```python
from build123d import *

# Parameters (mm, degrees)
F2_SIZE = 0.1


with BuildPart() as f1:
    # F0 (on Right) → F1 (revolve)
    with BuildSketch(Plane.YZ):
        Polygon((-21.5, 2.25), (0, 2.25), (0, 4.5), (-0.8, 4.5), (-0.8, 4), (-1.6, 4), (-1.6, 4.5), (-2.4, 4.5), (-2.4, 3.5), (-13.7, 3.5), (-13.7, 3), (-20.5, 3), (-21.5, 2.5), align=None)
    revolve(axis=Axis((0, -10.75, 0), (0, -1, 0)))

    # F2
    f2_edges = [f1.edges().sort_by_distance(p)[0] for p in [
        (0, -13.7, -3.5),
    ]]
    chamfer(f2_edges, length=F2_SIZE)


solid = f1.part
```
Work out the finished part from the listing and answer in its coordinate system (mm). A direction names the side the tool comes from. Coordinates: 2 decimals unless noted, no trailing zeros. Write each loop counter-clockwise with the first axis right and the second up, starting at its lowest first coordinate (ties: lowest second). Pieces come first, ordered by that corner, then holes. Notation, with made-up numbers: (83.5, -30) - (130.5, -30) arc R14 ccw to (130.5, -17) - close; hole circle Ø2 at (73.25, 57.5). An arc over 180 degrees is marked (long way). Answer as a JSON object with one key per item and string values.
Q1. Which of the six approach directions +Z, -Z, +X, -X, +Y, -Y give full straight-line access (tool end or side, diameter ignored) to faces 1 (the cylindrical face through (0, -17, -3)), 2 (the flat face through (3, -1.6, 3)), 3 (the cylindrical face through (-4.46, -0.41, -0.59))?
Results list:
{"face 1": "-Y", "face 2": "none", "face 3": "+Y, -Y"}
Q2. Given pin 1 Ø1.5 at (x, z) = (3, 2) entering from -Y; pin 2 Ø1.5 at (y, z) = (-3.5, 0.5) entering from -X; pin 3 Ø4.5 at (x, z) = (-0.5, 2) entering from -Y; pin 4 Ø1.5 at (y, z) = (-13, 3) entering from +X, each flat-ended and moving along its own axis, determine where each tip first touches the part or whether it passes through.
Results list:
{"pin 1": "stops at y = -20.79", "pin 2": "stops at x = -3.5", "pin 3": "stops at y = -21.5", "pin 4": "stops at x = 2.68"}
Q3. For a pull along Z with two mould halves and no side action, classify faces 4 (the cylindrical face through (-4.46, -2.01, -0.59)), 5 (the flat face through (4, -2.4, 0)), 6 (the cylindrical face through (-2.23, -10.6, -0.29)) as pulls with the +Z half, pulls with the -Z half, needs draft (parallel to the pull), parting line crosses it, or undercut.
Results list:
{"face 4": "parting line crosses it", "face 5": "needs draft", "face 6": "undercut"}
Q4. Find section B-B (y = -7.25). Write down the section's boundary in (x, z), plus the area to 3 significant figures.
Results list:
{"outline": "circle Ø7 at (0, 0); hole circle Ø4.5 at (0, 0)", "area": "22.6 mm^2"}
Q5. Consider L1, parallel to Y at x = -2.75, z = 3.5; L2, parallel to X at y = -8.5, z = 0; L3, parallel to X at y = -16.75, z = 0. Determine where each line is inside the solid, lowest interval first. Write a range as from..to.
Results list:
{"L1": "y = -2.4..-1.6, -0.8..0", "L2": "x = -3.5..-2.25, 2.25..3.5", "L3": "x = -3..-2.25, 2.25..3"}
Q6. Find section C-C (y = -2). Write down the section's boundary in (x, z).
Results list:
{"outline": "circle Ø9 at (0, 0); hole circle Ø4.5 at (0, 0)"}
Q7. Find section A-A (z = 0). Write down the section's boundary in (x, y).
Results list:
{"outline": "(-4.5, -2.4) - (-3.5, -2.4) - (-3.5, -13.6) - (-3.4, -13.7) - (-3, -13.7) - (-3, -20.5) - (-2.5, -21.5) - (-2.25, -21.5) - (-2.25, 0) - (-4.5, 0) - (-4.5, -0.8) - (-4, -0.8) - (-4, -1.6) - (-4.5, -1.6) - close; (2.25, -21.5) - (2.5, -21.5) - (3, -20.5) - (3, -13.7) - (3.4, -13.7) - (3.5, -13.6) - (3.5, -2.4) - (4.5, -2.4) - (4.5, -1.6) - (4, -1.6) - (4, -0.8) - (4.5, -0.8) - (4.5, 0) - (2.25, 0) - close"}
